Can you work these out from the model? Positions are in its coordinate system, mm. Face numbers are marked on the shaded views. A direction names the side the tool comes from. Give positions to 0.01 mm unless a question says otherwise; leave off trailing zeros. Order: outer loops, then holes, each group sorted by start corner. A loop starts at its lowest first (then second) coordinate and runs counter-clockwise, first axis right, second up. Notation, with made-up numbers: (-27.5, 10) - (23.5, 10) arc R25 cw to (23.5, 27) - close; hole circle Ø3 at (76.25, 81). An arc over 180 degrees is marked (long way). Answer as a JSON object with one key per item and string values.
```python
from build123d import *

# Parameters (mm, degrees)
SKETCH1_W                        = 60
SKETCH1_H                        = 60
BOSS_EXTRUDE1_DEPTH              = 6.35
SKETCH2_W                        = 28
SKETCH2_H                        = 16
CUT_EXTRUDE1_DEPTH               = 43.898980174
CBORE_FOR_M2_5_SHCS1_D           = 3.1
CBORE_FOR_M2_5_SHCS1_CBORE_D     = 5.5
CBORE_FOR_M2_5_SHCS1_CBORE_DEPTH = 2.5
MOVE_FACE2_BY                    = 0.15
MOVE_FACE2_2_BY                  = 0.15
MOVE_FACE2_3_BY                  = 0.15
MOVE_FACE2_4_BY                  = 0.15
SKETCH5_W                        = 6.35
SKETCH5_H                        = 15
CUT_EXTRUDE2_DEPTH               = 43.898980174
CUT_EXTRUDE3_DEPTH               = 43.898980174
MIRROR2_COPY_1_DEPTH             = 43.898980174
FILLET1_R                        = 2


with BuildPart() as part:
    # Sketch1 → Boss-Extrude1 (new body)
    with BuildSketch(Plane(origin=(0, 0, 0), x_dir=(1, 0, 0), z_dir=(0, 1, 0))):
        Rectangle(SKETCH1_W, SKETCH1_H)
    extrude(amount=BOSS_EXTRUDE1_DEPTH)

    # Sketch2 → Cut-Extrude1 (cut, through all)
    with BuildSketch(Plane(origin=(0, 6.35, 0), x_dir=(1, 0, 0), z_dir=(0, 1, 0))):
        Rectangle(SKETCH2_W, SKETCH2_H)
    extrude(amount=-CUT_EXTRUDE1_DEPTH, mode=Mode.SUBTRACT)

    # CBORE for M2.5 SHCS1 (through all)
    with Locations(Plane(origin=(0, 0, 0), x_dir=(-1, 0, 0), z_dir=(0, -1, 0))):
        with Locations((-11, 20), (11, 20), (-11, -20), (11, -20)):
            CounterBoreHole(CBORE_FOR_M2_5_SHCS1_D / 2, CBORE_FOR_M2_5_SHCS1_CBORE_D / 2, CBORE_FOR_M2_5_SHCS1_CBORE_DEPTH)

    # Move Face2: a face moved outward by 0.15
    extrude(part.faces().sort_by_distance((11, 2.5, -17.8))[0], amount=MOVE_FACE2_BY, dir=(0, -1, 0))

    # Move Face2 2: a face moved outward by 0.15
    extrude(part.faces().sort_by_distance((11, 2.5, 22.2))[0], amount=MOVE_FACE2_2_BY, dir=(0, -1, 0))

    # Move Face2 3: a face moved outward by 0.15
    extrude(part.faces().sort_by_distance((-11, 2.5, 22.2))[0], amount=MOVE_FACE2_3_BY, dir=(0, -1, 0))

    # Move Face2 4: a face moved outward by 0.15
    extrude(part.faces().sort_by_distance((-11, 2.5, -17.8))[0], amount=MOVE_FACE2_4_BY, dir=(0, -1, 0))

    # Sketch5 → Cut-Extrude2 (cut, through all)
    with BuildSketch(Plane(origin=(0, 6.35, 0), x_dir=(1, 0, 0), z_dir=(0, 1, 0))):
        with Locations((21.825, 17.5)):
            Rectangle(SKETCH5_W, SKETCH5_H)
    extrude(amount=-CUT_EXTRUDE2_DEPTH, mode=Mode.SUBTRACT)

    # Sketch6 → Cut-Extrude3 (cut, through all)
    with BuildSketch(Plane(origin=(0, 6.35, 0), x_dir=(1, 0, 0), z_dir=(0, 1, 0))):
        with BuildLine():
            Line((23.267949192, 25), (20.382050808, 25))
            ThreePointArc((20.382050808, 25), (19.882050808, 25.133974596), (19.516025404, 25.5))
            ThreePointArc((19.516025404, 25.5), (17.942893219, 25.707106781), (18.15, 24.133974596))
            ThreePointArc((18.15, 24.133974596), (18.516025404, 23.767949192), (18.65, 23.267949192))
            Line((18.65, 23.267949192), (18.65, 11.732050808))
            ThreePointArc((18.65, 11.732050808), (18.516025404, 11.232050808), (18.15, 10.866025404))
            ThreePointArc((18.15, 10.866025404), (17.942893219, 9.292893219), (19.516025404, 9.5))
            ThreePointArc((19.516025404, 9.5), (19.882050808, 9.866025404), (20.382050808, 10))
            Line((20.382050808, 10), (23.267949192, 10))
            ThreePointArc((23.267949192, 10), (23.767949192, 9.866025404), (24.133974596, 9.5))
            ThreePointArc((24.133974596, 9.5), (25.707106781, 9.292893219), (25.5, 10.866025404))
            ThreePointArc((25.5, 10.866025404), (25.133974596, 11.232050808), (25, 11.732050808))
            Line((25, 11.732050808), (25, 23.267949192))
            ThreePointArc((25, 23.267949192), (25.133974596, 23.767949192), (25.5, 24.133974596))
            ThreePointArc((25.5, 24.133974596), (25.707106781, 25.707106781), (24.133974596, 25.5))
            ThreePointArc((24.133974596, 25.5), (23.767949192, 25.133974596), (23.267949192, 25))
        make_face()
    cut_extrude3 = extrude(amount=-CUT_EXTRUDE3_DEPTH, mode=Mode.SUBTRACT)

    # Mirror1: Cut-Extrude3 across plane
    add(cut_extrude3.mirror(Plane.XY), mode=Mode.SUBTRACT)

    # Mirror2: Cut-Extrude3 across plane
    add(cut_extrude3.mirror(Plane(origin=(0, 0, 0), x_dir=(0, 0, 1), z_dir=(1, 0, 0))), mode=Mode.SUBTRACT)

    # Mirror2 copy 1 sketch → Mirror2 copy 1 (cut, through all)
    with BuildSketch(Plane(origin=(0, 6.35, 0), x_dir=(-1, 0, 0), z_dir=(0, 1, 0))):
        with BuildLine():
            Line((23.267949192, 25), (20.382050808, 25))
            ThreePointArc((20.382050808, 25), (19.882050808, 25.133974596), (19.516025404, 25.5))
            ThreePointArc((19.516025404, 25.5), (17.942893219, 25.707106781), (18.15, 24.133974596))
            ThreePointArc((18.15, 24.133974596), (18.516025404, 23.767949192), (18.65, 23.267949192))
            Line((18.65, 23.267949192), (18.65, 11.732050808))
            ThreePointArc((18.65, 11.732050808), (18.516025404, 11.232050808), (18.15, 10.866025404))
            ThreePointArc((18.15, 10.866025404), (17.942893219, 9.292893219), (19.516025404, 9.5))
            ThreePointArc((19.516025404, 9.5), (19.882050808, 9.866025404), (20.382050808, 10))
            Line((20.382050808, 10), (23.267949192, 10))
            ThreePointArc((23.267949192, 10), (23.767949192, 9.866025404), (24.133974596, 9.5))
            ThreePointArc((24.133974596, 9.5), (25.707106781, 9.292893219), (25.5, 10.866025404))
            ThreePointArc((25.5, 10.866025404), (25.133974596, 11.232050808), (25, 11.732050808))
            Line((25, 11.732050808), (25, 23.267949192))
            ThreePointArc((25, 23.267949192), (25.133974596, 23.767949192), (25.5, 24.133974596))
            ThreePointArc((25.5, 24.133974596), (25.707106781, 25.707106781), (24.133974596, 25.5))
            ThreePointArc((24.133974596, 25.5), (23.767949192, 25.133974596), (23.267949192, 25))
        make_face()
    extrude(amount=-MIRROR2_COPY_1_DEPTH, mode=Mode.SUBTRACT)

    # Fillet1
    fillet1_edges = [part.edges().sort_by_distance(p)[0] for p in [
        (-14, 3.175, 8),
        (-14, 3.175, -8),
        (14, 3.175, -8),
        (14, 3.175, 8),
        (-30, 3.175, -30),
        (30, 3.175, -30),
        (30, 3.175, 30),
        (-30, 3.175, 30),
    ]]
    fillet(fillet1_edges, radius=FILLET1_R)


solid = part.part
```
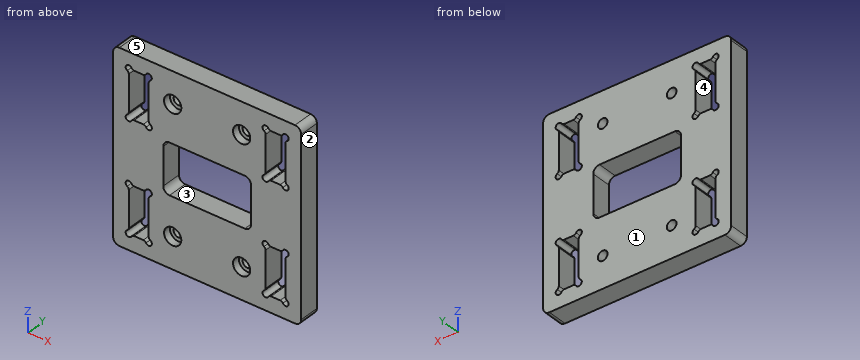
Q1. If we section it at C-C, the plane x = 11: Please give me the cut outline in (y, z), then the cut area to 3 significant figures.
Recorded:
{"outline": "(0, -30) - (6.35, -30) - (6.35, -21.55) - (2.35, -21.55) - (2.35, -22.75) - (0, -22.75) - close; (0, -17.25) - (2.35, -17.25) - (2.35, -18.45) - (6.35, -18.45) - (6.35, -8) - (0, -8) - close; (0, 8) - (6.35, 8) - (6.35, 18.45) - (2.35, 18.45) - (2.35, 17.25) - (0, 17.25) - close; (0, 22.75) - (2.35, 22.75) - (2.35, 21.55) - (6.35, 21.55) - (6.35, 30) - (0, 30) - close", "area": "229 mm^2"}
Q2. I'm going to push a flat-ended pin straight in: pin 1 Ø4.5 at (x, z) = (-11, 20) entering from -Y. Where does the tip first touch, or does it pass through?
Recorded:
{"pin 1": "stops at y = 2.35"}
Q3. We'd pull the mould along X, two halves only. Please class the marked faces 1, 2 and 3: released by +X, released by -X, zero draft, split by the parting line, or undercut.
Recorded:
{"face 1": "zero draft", "face 2": "released by +X", "face 3": "undercut"}
Q4. I need wall thicknesses on L1, parallel to Z at x = -11, y = 1.25; L2, parallel to X at y = 1.3, z = -20; L3, parallel to Z at x = 20.5, y = 3.5. Which ranges of each line are inside material? Lowest first, please.
Recorded:
{"L1": "z = -30 to -22.75, -17.25 to -8, 8 to 17.25, 22.75 to 30", "L2": "x = -30 to -25, -18.65 to -13.75, -8.25 to 8.25, 13.75 to 18.65, 25 to 30", "L3": "z = -30 to -25, -10 to 10, 25 to 30"}
Q5. Which directions (+Z, -Z, +X, -X, +Y, -Y) give clear straight access to the entire face, cutting with the end or side of a thin tool? Please do the marked faces 4 and 5.
Recorded:
{"face 4": "+Y, -Y", "face 5": "+Z, +X, -X, +Y, -Y"}
Q6. If we section it at B-B, the plane z = 7: Please give me the cut outline in (x, y), then the cut area to 3 significant figures.
Recorded:
{"outline": "(-30, 0) - (-13.73, 0) - (-13.73, 6.35) - (-30, 6.35) - close; (13.73, 0) - (30, 0) - (30, 6.35) - (13.73, 6.35) - close", "area": "207 mm^2"}
Q7. If we section it at A-A, the plane x = 3: Please give me the cut outline in (y, z), then the cut area to 3 significant figures.
Recorded:
{"outline": "(0, -30) - (6.35, -30) - (6.35, -8) - (0, -8) - close; (0, 8) - (6.35, 8) - (6.35, 30) - (0, 30) - close", "area": "279 mm^2"}
Q8. If we section it at D-D, the plane y = 1.25: Count the separate pieces of the cut face and the enclosed holes in it, then the cut area to 3 significant figures.
Recorded:
{"separate pieces": "1", "enclosed holes": "9", "area": "2,640 mm^2"}
